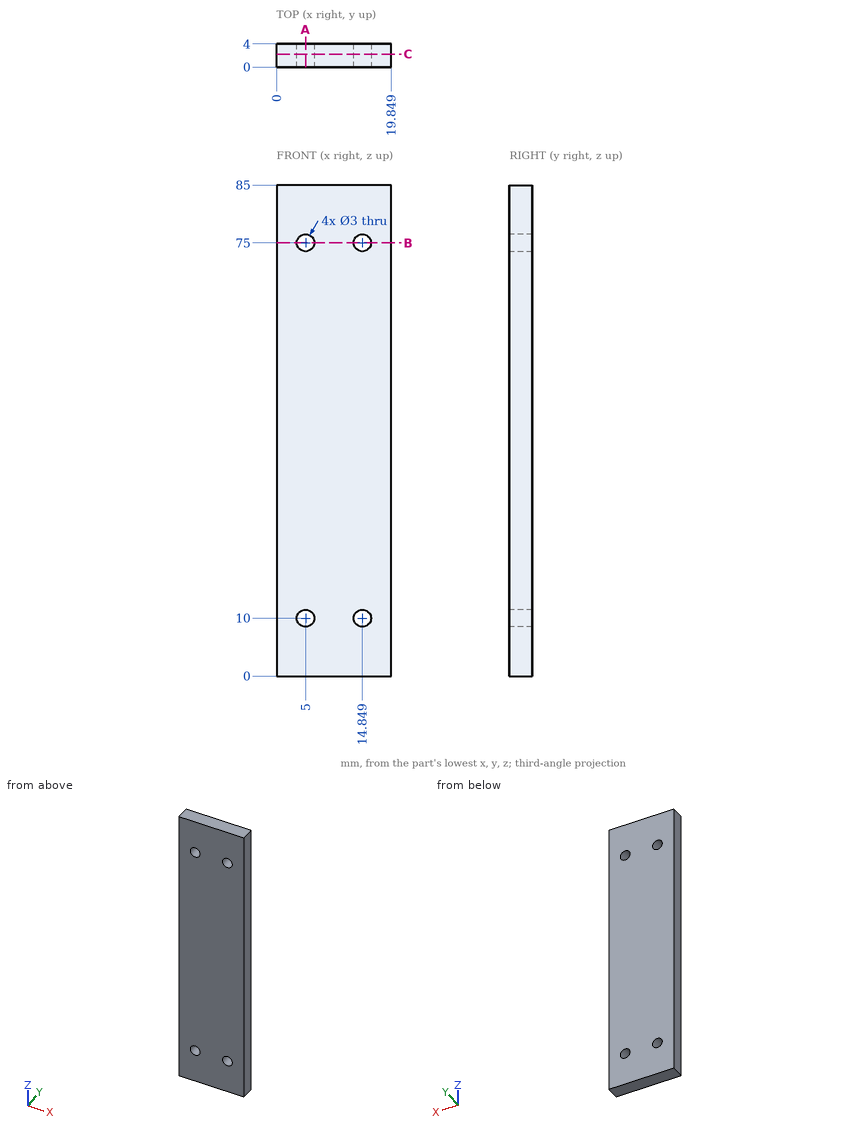
The figure shows three views and two pictorial views of one solid part (mm, origin at its lowest corner). Answer the questions. Give positions to 0.01 mm unless a question says otherwise; leave off trailing zeros. Loops run counter-clockwise (first coordinate to the right, second up) from the corner with the lowest first, then second, coordinate; pieces in that order, holes last. Notation, with made-up numbers: (45.25, -12) -> (86.25, -12) arc R21 ccw to (86.25, -7) -> close; hole circle Ø1 at (46.25, -9.75). An arc over 180 degrees is marked (long way). Use a Markdown table: item, result. Add a question column.
1. A flat-ended cylindrical pin translates along its axis: pin 1 Ø2.5 at (x, z) = (5, 10) entering from +Y. Find the tip coordinate at first contact, or state that the pin passes through.
2. Section B-B on z = 75 is taken. Determine the outline of the cut face in (x, y).
3. Section A-A on x = 5 is taken. Determine the outline of the cut face in (y, z).
4. Find the intervals of material crossed by probe 1 along Z at (x, y) = (5, 2.4); probe 2 along Z at (x, y) = (4.25, 3.45); probe 3 along X at (y, z) = (2.3, 11), in increasing order.
5. Section C-C on y = 2.25 is taken. Determine the outline of the cut face in (x, z), and give its area (3 significant figures).
Results below:
| question | item | result |
|---|---|---|
| 1 | pin 1 | passes through |
| 2 | outline | (0, 0) -> (3.5, 0) -> (3.5, 4) -> (0, 4) -> close; (6.5, 0) -> (13.35, 0) -> (13.35, 4) -> (6.5, 4) -> close; (16.35, 0) -> (19.85, 0) -> (19.85, 4) -> (16.35, 4) -> close |
| 3 | outline | (0, 0) -> (4, 0) -> (4, 8.5) -> (0, 8.5) -> close; (0, 11.5) -> (4, 11.5) -> (4, 73.5) -> (0, 73.5) -> close; (0, 76.5) -> (4, 76.5) -> (4, 85) -> (0, 85) -> close |
| 4 | probe 1 | z = 0 to 8.5, 11.5 to 73.5, 76.5 to 85 |
| 4 | probe 2 | z = 0 to 8.7, 11.3 to 73.7, 76.3 to 85 |
| 4 | probe 3 | x = 0 to 3.88, 6.12 to 13.73, 15.97 to 19.85 |
| 5 | outline | (0, 0) -> (19.85, 0) -> (19.85, 85) -> (0, 85) -> close; hole circle Ø3 at (5, 10); hole circle Ø3 at (5, 75); hole circle Ø3 at (14.85, 10); hole circle Ø3 at (14.85, 75) |
| 5 | area | 1,660 mm^2 |
